```python
from build123d import *

# Parameters (mm, degrees)
SKETCH5_R                = 140
SKETCH5_R_2              = 97
BOSS_EXTRUDE2_DEPTH      = 225
SKETCH6_R                = 23.5
BOSS_EXTRUDE3_DEPTH      = 32
CIRPATTERN1_COUNT        = 3
MIRROR1_COPY_1_SKETCH_R  = 23.5
MIRROR1_COPY_1_DEPTH     = 32
MIRROR1_COPY_2_SKETCH_R  = 23.5
MIRROR1_COPY_2_DEPTH     = 32
BOSS_EXTRUDE4_REACH      = 491.361
BOSS_EXTRUDE4_END_RADIUS = 140
SKETCH7_R                = 100
SKETCH9_R                = 50
CUT_EXTRUDE2_DEPTH       = 25
SKETCH10_R               = 25
CUT_EXTRUDE3_DEPTH       = 470.945957604
SKETCH11_R               = 12
CUT_EXTRUDE4_DEPTH       = 15
CIRPATTERN4_COUNT        = 3


with BuildPart() as part:
    # Sketch5 → Boss-Extrude2 (new body)
    with BuildSketch(Plane.XY):
        Circle(SKETCH5_R)
        Circle(SKETCH5_R_2, mode=Mode.SUBTRACT)
    extrude(amount=BOSS_EXTRUDE2_DEPTH)

    # Sketch6 → Boss-Extrude3 (add)
    with BuildSketch(Plane.XY.offset(225)):
        with BuildLine():
            Line((50, 105.027441764), (-50, 105.027441764))
            Line((-50, 105.027441764), (-50, 174.972558236))
            ThreePointArc((-50, 174.972558236), (0, 225.000007531), (50, 174.972558236))
            Line((50, 174.972558236), (50, 105.027441764))
        make_face()
        with Locations((0, 175)):
            Circle(SKETCH6_R, mode=Mode.SUBTRACT)
    boss_extrude3 = extrude(amount=-BOSS_EXTRUDE3_DEPTH)

    # CirPattern1: Boss-Extrude3 ×3 about axis
    cirpattern1_axis = Axis((0, 0, 0), (0, 0, 1))
    for i in range(1, CIRPATTERN1_COUNT):
        add(boss_extrude3.rotate(cirpattern1_axis, i * 360 / CIRPATTERN1_COUNT))

    # Mirror1: Boss-Extrude3 across plane
    add(boss_extrude3.mirror(Plane(origin=(0, 0, 112.5), x_dir=(1, 0, 0), z_dir=(0, 0, -1))))

    # Mirror1 copy 1 sketch → Mirror1 copy 1 (add)
    with BuildSketch(Plane(origin=(0, 0, 0), x_dir=(-0.4999999999999998, 0.8660254037844387, 0), z_dir=(0, 0, -1))):
        with BuildLine():
            Line((50, -105.027441764), (-50, -105.027441764))
            Line((-50, -105.027441764), (-50, -174.972558236))
            ThreePointArc((-50, -174.972558236), (0, -225.000007531), (50, -174.972558236))
            Line((50, -174.972558236), (50, -105.027441764))
        make_face()
        with Locations((0, -175)):
            Circle(MIRROR1_COPY_1_SKETCH_R, mode=Mode.SUBTRACT)
    extrude(amount=-MIRROR1_COPY_1_DEPTH)

    # Mirror1 copy 2 sketch → Mirror1 copy 2 (add)
    with BuildSketch(Plane(origin=(0, 0, 0), x_dir=(-0.5000000000000004, -0.8660254037844384, 0), z_dir=(0, 0, -1))):
        with BuildLine():
            Line((50, -105.027441764), (-50, -105.027441764))
            Line((-50, -105.027441764), (-50, -174.972558236))
            ThreePointArc((-50, -174.972558236), (0, -225.000007531), (50, -174.972558236))
            Line((50, -174.972558236), (50, -105.027441764))
        make_face()
        with Locations((0, -175)):
            Circle(MIRROR1_COPY_2_SKETCH_R, mode=Mode.SUBTRACT)
    extrude(amount=-MIRROR1_COPY_2_DEPTH)

    # Boss-Extrude4: up to this cylinder (the profile starts outside it)
    boss_extrude4_end = Plane(origin=(0, 0, 112.5), z_dir=(0, 0, -1)) * Cylinder(BOSS_EXTRUDE4_END_RADIUS, 1263.722, mode=Mode.PRIVATE)
    # Sketch7 → Boss-Extrude4 (add, up to the surface)
    with BuildSketch(Plane(origin=(0, -160, 0), x_dir=(1, 0, 0), z_dir=(0, 1, 0)), mode=Mode.PRIVATE) as boss_extrude4_sk1:
        with Locations(Location((0, -112.5, 0), (0, 0, 90))):
            Circle(SKETCH7_R)
    boss_extrude4_tool1 = extrude(boss_extrude4_sk1.sketch, amount=BOSS_EXTRUDE4_REACH, mode=Mode.PRIVATE) - boss_extrude4_end
    add(boss_extrude4_tool1.solids().sort_by_distance((0, -160, 112.5))[0])

    # Sketch9 → Cut-Extrude2 (cut)
    with BuildSketch(Plane.XZ.offset(160)):
        with Locations(Location((0, 112.5, 0), (0, 0, 270))):
            Circle(SKETCH9_R)
    extrude(amount=-CUT_EXTRUDE2_DEPTH, mode=Mode.SUBTRACT)

    # Sketch10 → Cut-Extrude3 (cut, through all)
    with BuildSketch(Plane.XZ.offset(135)):
        with Locations(Location((0, 112.5, 0), (0, 0, 270))):
            Circle(SKETCH10_R)
    extrude(amount=-CUT_EXTRUDE3_DEPTH, mode=Mode.SUBTRACT)

    # Sketch11 → Cut-Extrude4 (cut)
    with BuildSketch(Plane.XZ.offset(160)):
        with Locations(Location((0, 187.5, 0), (0, 0, 270))):
            Circle(SKETCH11_R)
    cut_extrude4 = extrude(amount=-CUT_EXTRUDE4_DEPTH, mode=Mode.SUBTRACT)

    # CirPattern4: Cut-Extrude4 ×3 about axis
    cirpattern4_axis = Axis((0, 0, 112.5), (0, 1, 0))
    for i in range(1, CIRPATTERN4_COUNT):
        add(cut_extrude4.rotate(cirpattern4_axis, i * 360 / CIRPATTERN4_COUNT), mode=Mode.SUBTRACT)


solid = part.part
```
Geometry check sheet. Reference: the model listing, model coordinates, mm. A direction names the side the tool comes from. Round coordinates to 2 decimals unless told otherwise and drop trailing zeros. Write each loop counter-clockwise with the first axis right and the second up, starting at its lowest first coordinate (ties: lowest second). Pieces come first, ordered by that corner, then holes. Notation, with made-up numbers: (43, 13) -> (53, 13) arc R28 ccw to (53, 50) -> close; hole circle Ø9 at (37.5, -27.75). An arc over 180 degrees is marked (long way). Put each result on its own line as item: value.
1) Cross-section at B-B, the plane z = 75. Enter the section's corners in (x, y), plus the area to 3 significant figures.
Recorded:
outline: (-92.7, -160) -> (-76.95, -160) -> (-76.95, -145) -> (-52.95, -145) -> (-52.95, -160) -> (-33.07, -160) -> (-33.07, -135) -> (33.07, -135) -> (33.07, -160) -> (52.95, -160) -> (52.95, -145) -> (76.95, -145) -> (76.95, -160) -> (92.7, -160) -> (92.7, -104.91) arc R140 ccw (long way) to (-92.7, -104.91) -> close; hole circle Ø194 at (0, 0)
area: 35,400 mm2
2) Thickness scan on probe 1 along Z at (x, y) = (141, -121); probe 2 along Y at (x, z) = (2, 75); probe 3 along X at (y, z) = (-87, 8). Record the ranges inside material, lowest first. Write a range as from..to.
Recorded:
probe 1: z = 0..32, 193..225
probe 2: y = -135..-96.98, 96.98..139.99
probe 3: x = -201.55..-175.05, -128.06..-42.9, 42.9..128.06, 175.05..201.55
3) Access from +Z, -Z, +X, -X, +Y, -Y to the whole of each face (thin tool, end or side, straight path). Record for faces 1 (the face through (-3.06, 198.3, 209.22)), 2 (the face through (-173, -99, 193)), 3 (the face through (-65, -145, 75)).
Recorded:
face 1: +Z, -Z
face 2: -X, -Y
face 3: -Y
4) Cross-section at D-D, the plane y = -87.5. Give the number of separate pieces and of enclosed holes in the cut face, plus the area to 3 significant figures.
Recorded:
separate pieces: 6
enclosed holes: 0
area: 36,100 mm2
5) Release check for a two-part mould opening along Y. For faces 4 (the face through (-50, 153, 16)), 5 (the face through (195.395, -111.541, 15.776)), 6 (the face through (-175.03, -88.53, 15.78)), 7 (the face through (-107.12, -119.58, 15.78)) record: pulls with the +Y half, pulls with the -Y half, needs draft (parallel to the pull), parting line crosses it, or undercut.
Recorded:
face 4: needs draft
face 5: parting line crosses it
face 6: undercut
face 7: pulls with the -Y half
6) Cross-section at A-A, the plane y = 0. Enter the section's corners in (x, z), plus the area to 4 significant figures.
Recorded:
outline: (-140, 0) -> (-97, 0) -> (-97, 225) -> (-140, 225) -> close; (97, 0) -> (140, 0) -> (140, 225) -> (97, 225) -> close
area: 19,350 mm2
7) Cross-section at C-C, the plane z = 121.5. Enter the section's corners in (x, y).
Recorded:
outline: (-99.59, -160) -> (-49.18, -160) -> (-49.18, -135) -> (-23.32, -135) -> (-23.32, -94.15) arc R97 cw to (-23.32, 94.15) -> (-23.32, 138.04) arc R140 ccw to (-99.59, -98.39) -> close; (23.32, -135) -> (49.18, -135) -> (49.18, -160) -> (99.59, -160) -> (99.59, -98.39) arc R140 ccw to (23.32, 138.04) -> (23.32, 94.15) arc R97 cw to (23.32, -94.15) -> close
8) Depth check by flat-ended pin: P1, Ø6, axis at y = 125.5, z = 126, coming from the +X side; P2, Ø6, axis at y = 42, z = 106.5, coming from the +X side; P3, Ø5, axis at y = 43.5, z = 72, coming from the -X side. Enter the tip coordinate at first touch or a pass-through.
Recorded:
P1: stops at x = 67.78
P2: stops at x = 134.46
P3: stops at x = -133.86
